Geometry: final body of the model. Coordinates: model frame, mm. A direction names the side the tool comes from. Round coordinates to 2 decimals unless told otherwise and drop trailing zeros. Order: outer loops, then holes, each group sorted by start corner. A loop starts at its lowest first (then second) coordinate and runs counter-clockwise, first axis right, second up. Notation, with made-up numbers: (-19, 22.5) - (7, 22.5) arc R20 ccw to (7, 58.5) - close; hole circle Ø2 at (63, -0.75). An arc over 180 degrees is marked (long way). Put each result on its own line as item: value. Start each with the question number.
(1) Pin query (flat end, axial travel): P1, Ø2, axis at x = -1.5, z = 5, coming from the +Y side; P2, Ø5, axis at x = 4.5, y = -13, coming from the -Z side; P3, Ø3, axis at y = -7.5, z = 4, coming from the -X side; P4, Ø2, axis at y = 27.5, z = 2, coming from the -X side. Return the tip coordinate at first contact, or that it passes through.
(2) Access query for faces 4 (the face through (9, 7, 7)), 5 (the face through (-29.008, -21.724, 3.451)). Directions: +Z, -Z, +X, -X, +Y, -Y. A direction counts if a zero-diameter tool reaches every point of the face in a straight line with its end or side. Return the directions, or none.
(3) Pull-direction query (X, two-part tool) for faces 1 (the face through (0.48, 43.65, 3.45)), 2 (the face through (33.318, -14, 3)), 3 (the face through (9, 7, 0)); classes: released by +X, released by -X, zero draft, split by the parting line, or undercut.
(4) Section B-B (x = 20). Output: boundary loops of the cut face in (y, z), and give its area (3 significant figures).
(5) Section D-D (x = 2). Output: boundary loops of the cut face in (y, z).
(6) Material intervals for L1, parallel to Y at x = 0, z = 1.75; L2, parallel to X at y = -11, z = 6.5; L3, parallel to Y at x = 9.5, z = 1.25, sorted ascending. Write a range as [from, to].
(7) Section A-A (y = -16). Output: boundary loops of the cut face in (x, z).
(8) Section C-C (y = 31.5). Output: boundary loops of the cut face in (x, z).
from build123d import *

# Parameters (mm, degrees)
F0_R     = 10.9
F1_DEPTH = 7


with BuildPart() as f1:
    # F0 (on Top) → F1 (new body)
    with BuildSketch(Plane.XY):
        with BuildLine():
            ThreePointArc((21.619418, 0.541571), (18.675118, 10.905618), (11.095609, 18.562866))
            ThreePointArc((11.095609, 18.562866), (0, 43.656797), (-11.095609, 18.562866))
            ThreePointArc((-11.095609, 18.562866), (-18.833376, 10.629979), (-21.625995, -0.094059))
            ThreePointArc((-21.625995, -0.094059), (-37.738757, -22.402484), (-10.438593, -18.940124))
            ThreePointArc((-10.438593, -18.940124), (0.363458, -21.623146), (11.069236, -18.578605))
            ThreePointArc((11.069236, -18.578605), (38.482629, -21.234049), (21.619418, 0.541571))
        make_face()
        Polygon((-16.317514, -19.235876), (-24.817514, -24.143353), (-33.317514, -19.235876), (-33.317514, -9.420921), (-24.817514, -4.513444), (-16.317514, -9.420921), align=None, mode=Mode.SUBTRACT)
        Circle(F0_R, mode=Mode.SUBTRACT)
        Polygon((24.817514, -4.513444), (33.317514, -9.420921), (33.317514, -19.235876), (24.817514, -24.143353), (16.317514, -19.235876), (16.317514, -9.420921), align=None, mode=Mode.SUBTRACT)
        Polygon((0, 38.471752), (8.5, 33.564274), (8.5, 23.74932), (0, 18.841842), (-8.5, 23.74932), (-8.5, 33.564274), align=None, mode=Mode.SUBTRACT)
    extrude(amount=F1_DEPTH)


solid = f1.part
Checks:
1. P1: stops at y = 43.65
1. P2: stops at z = 0
1. P3: stops at x = -38.7
1. P4: stops at x = -15
2. face 4: +Z, +X, -X, +Y, -Y
2. face 5: +Z, -Z
3. face 1: split by the parting line
3. face 2: undercut
3. face 3: zero draft
4. outline: (-28, 0) - (-21.36, 0) - (-21.36, 7) - (-28, 7) - close; (-7.29, 0) - (8.23, 0) - (8.23, 7) - (-7.29, 7) - close
4. area: 155 mm²
5. outline: (-21.53, 0) - (-10.71, 0) - (-10.71, 7) - (-21.53, 7) - close; (10.71, 0) - (20, 0) - (20, 7) - (10.71, 7) - close; (37.32, 0) - (43.52, 0) - (43.52, 7) - (37.32, 7) - close
6. L1: y = [-21.63, -10.9], [10.9, 18.84], [38.47, 43.66]
6. L2: x = [-39.37, -33.32], [-16.32, 16.32], [33.32, 40.05]
6. L3: y = [-19.43, -5.34], [5.34, 40.26]
7. outline: (-39.79, 0) - (-33.32, 0) - (-33.32, 7) - (-39.79, 7) - close; (-16.32, 0) - (16.32, 0) - (16.32, 7) - (-16.32, 7) - close; (33.32, 0) - (40.21, 0) - (40.21, 7) - (33.32, 7) - close
8. outline: (-14.73, 0) - (-8.5, 0) - (-8.5, 7) - (-14.73, 7) - close; (8.5, 0) - (14.73, 0) - (14.73, 7) - (8.5, 7) - close
